Source: CAD feature listing. Evaluate the final solid. Frame: model axes, mm. Face numbers are marked on the shaded views. A direction names the side the tool comes from. Give positions to 0.01 mm unless a question says otherwise; leave off trailing zeros. Loops run counter-clockwise (first coordinate to the right, second up) from the corner with the lowest first, then second, coordinate; pieces in that order, holes last.
from build123d import *

# Parameters (mm, degrees)
BOSS_EXTRUDE1_DEPTH = 100
SKETCH2_R           = 3.175
CUT_EXTRUDE1_DEPTH  = 182.919520377


with BuildPart() as part:
    # Sketch1 → Boss-Extrude1 (new body)
    with BuildSketch(Plane(origin=(0, 0, 0), x_dir=(0, 0, -1), z_dir=(1, 0, 0))):
        Polygon((0, 0), (-25, 43.301270189), (-20.669872981, 45.801270189), (2.886751346, 5), (150, 5), (150, 0), align=None)
    extrude(amount=BOSS_EXTRUDE1_DEPTH)

    # Sketch2 → Cut-Extrude1 (cut, through all)
    with BuildSketch(Plane(origin=(0, 2.5, -4.330127019), x_dir=(-1, 0, 0), z_dir=(0, 0.49999999999999806, -0.8660254037844397))):
        with Locations(Location((-75, 27.886751346, 0), (0, 0, 90))):
            Circle(SKETCH2_R)
        with Locations(Location((-50, 27.886751346, 0), (0, 0, 90))):
            Circle(SKETCH2_R)
    extrude(amount=-CUT_EXTRUDE1_DEPTH, mode=Mode.SUBTRACT)


solid = part.part
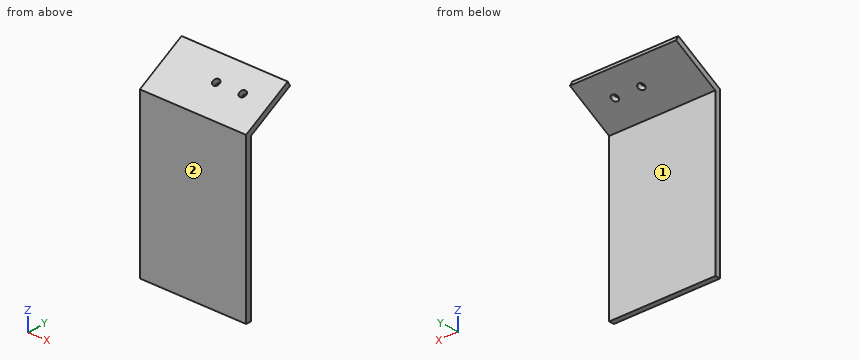
1) Cut plane B-B (z = -17). Return loops of the section in (x, y), and give its area (3 significant figures).
Checks:
outline: (0, 0) - (100, 0) - (100, 5) - (0, 5) - close
area: 500 mm2
2) Cut plane A-A (x = 40). Return loops of the section in (y, z).
Checks:
outline: (0, -150) - (5, -150) - (5, -2.89) - (45.8, 20.67) - (43.3, 25) - (0, 0) - close
3) Cut plane D-D (y = 15). Return loops of the section in (x, z), and give its area (3 significant figures).
Checks:
outline: (0, 2.89) - (100, 2.89) - (100, 8.66) - (0, 8.66) - close
area: 577 mm2
4) Cut plane C-C (y = 25). State how many separate pieces and enclosed holes the cut face has, and give its area (3 significant figures).
Checks:
separate pieces: 3
enclosed holes: 0
area: 508 mm2
5) Reachability of the marked faces 1 and 2 from +Z, -Z, +X, -X, +Y, -Y: full face, straight path, thin tool, end or side. Return the list, or none.
Checks:
face 1: -Z, +X, -X, +Y
face 2: +Z, -Z, +X, -X, -Y
6) Contact query for flat-ended pins moving along their axis: P1, Ø4, axis at x = 53, y = 33.5, coming from the -Z side; P2, Ø5, axis at x = 22.5, z = -132.5, coming from the +Y side; P3, Ø8, axis at x = 73, y = 30.5, coming from the +Z side. Output: stop coordinate, or through.
Checks:
P1: stops at z = 12.41
P2: stops at y = 5
P3: stops at z = 19.92
7) Ray query, probe 1 along Y at (x, z) = (27.5, -141); probe 2 along Z at (x, y) = (12, 34.5); probe 3 along Z at (x, y) = (67, 29.5). Return the intervals inside material, ascending.
Checks:
probe 1: y = 0 to 5
probe 2: z = 14.15 to 19.92
probe 3: z = 11.26 to 17.03
